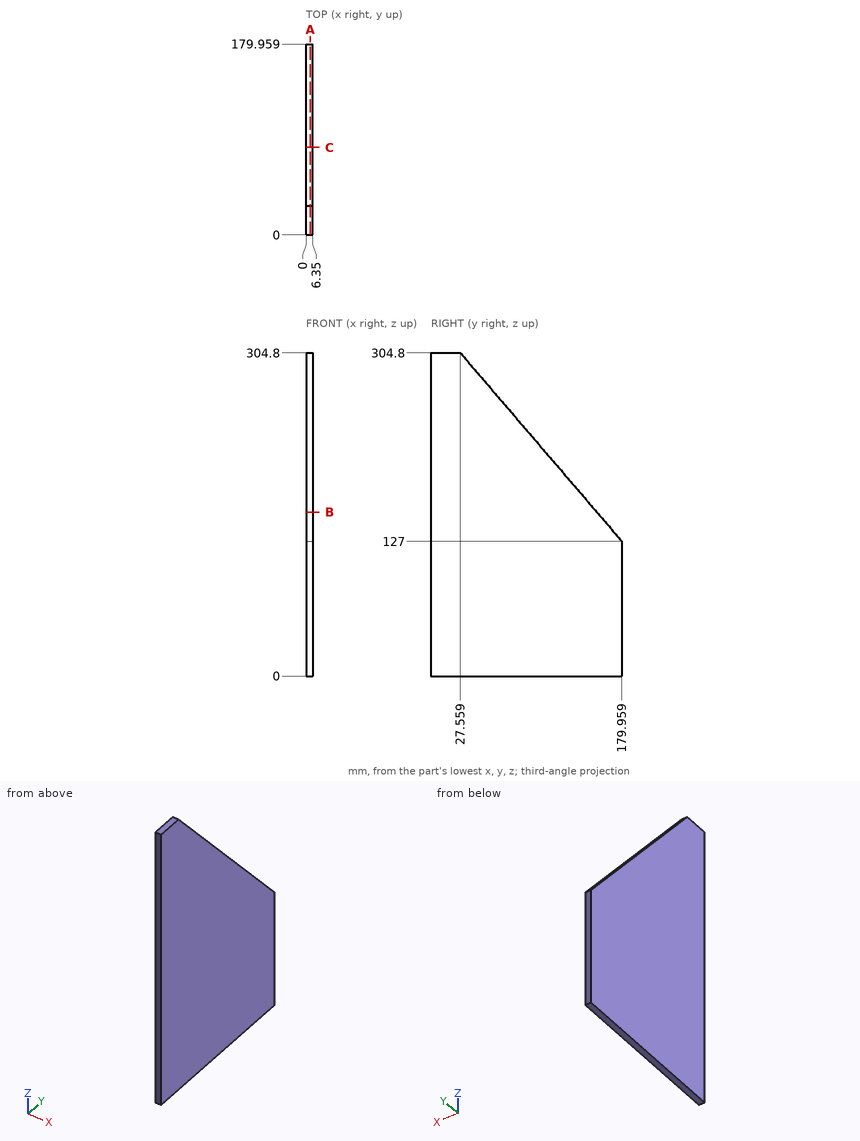
Part print with two shaded views. Sizes in mm from the minimum x, y, z corner. Give positions to 0.01 mm unless a question says otherwise; leave off trailing zeros. Order: outer loops, then holes, each group sorted by start corner. A loop starts at its lowest first (then second) coordinate and runs counter-clockwise, first axis right, second up. Notation, with made-up numbers: M -31.75,89 L 24.25,89 A10 cw 24.25,97 Z; hole C 48.25,46 d4. An arc over 180 degrees is marked long. Put each result on its own line as item: value.
Item 1: Drop a flat-ended pin along its axis: pin 1 Ø3 at (x, z) = (3.5, 179) entering from +Y. Give the stop position or say it passes through.
Results are:
pin 1: y = 136.67
Item 2: Cut at A-A on x = 4. Write the cut outline in (y, z), then the cut area to 3 significant figures.
Results are:
outline: M 0,0 L 179.96,0 L 179.96,127 L 27.56,304.8 L 0,304.8 Z
area: 41,300 mm2
Item 3: Cut at C-C on y = 82.5. Write the cut outline in (x, z).
Results are:
outline: M 0,0 L 6.35,0 L 6.35,240.7 L 0,240.7 Z
Item 4: Wall check: probe 1 along Y at (x, z) = (1.25, 151.5); probe 2 along Z at (x, y) = (1.5, 92.5); probe 3 along Y at (x, z) = (2.5, 283). Give the ranges that are in metal, low to high.
Results are:
probe 1: 0 to 158.96
probe 2: 0 to 229.04
probe 3: 0 to 46.24
Item 5: Cut at B-B on z = 154.5. Write the cut outline in (x, y), then the cut area to 3 significant figures.
Results are:
outline: M 0,0 L 6.35,0 L 6.35,156.39 L 0,156.39 Z
area: 993 mm2
